Can you work these out from the drawing? Everything is in mm from the part's minimum corner. A direction names the side the tool comes from. Coordinates: 2 decimals unless noted, no trailing zeros. Write each loop counter-clockwise with the first axis right and the second up, starting at its lowest first coordinate (ties: lowest second). Pieces come first, ordered by that corner, then holes. Notation, with made-up numbers: M 69,37.5 L 123,37.5 A25 cw 123,52.5 Z; hole C 74.5,55.5 d4. An arc over 180 degrees is marked long. Write item = value, one per line.
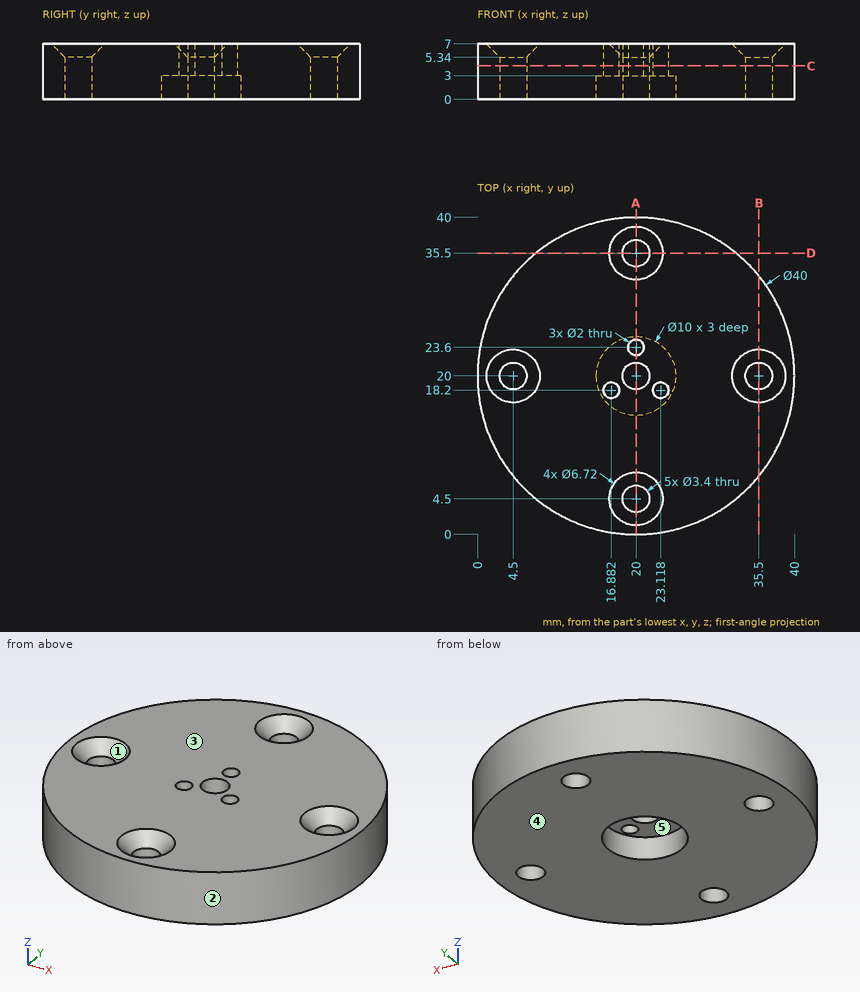
Item 1: Imagine slicing it at C-C (z = 4.25). State how many separate pieces and enclosed holes the cut face has, and give its area (3 significant figures).
Numbers:
separate_pieces = 1
enclosed_holes = 8
area = 1,200 mm²
Item 2: Imagine slicing it at B-B (x = 35.5). Write out the boundary of the cut face in (y, z).
Numbers:
outline = M 7.36,0 L 18.3,0 L 18.3,5.34 L 16.64,7 L 7.36,7 Z; M 21.7,0 L 32.64,0 L 32.64,7 L 23.36,7 L 21.7,5.34 Z
Item 3: If we mould it in two halves opening along Y, with no side actions, what happens to the marked faces 1, 2 and 3? For each: pulls with the +Y half, pulls with the -Y half, needs draft (parallel to the pull), parting line crosses it, or undercut.
Numbers:
face_1 = undercut
face_2 = parting line crosses it
face_3 = needs draft
Item 4: I'm going to push flat-ended pins straight in: P1, Ø4, axis at y = 15, z = 2, coming from the +X side; P2, Ø1, axis at x = 28, z = 3.5, coming from the +Y side. Where does each tip first touch, or does it pass through?
Numbers:
P1 = 39.77
P2 = 38.54
Item 5: Imagine slicing it at A-A (x = 20). Write out the boundary of the cut face in (y, z).
Numbers:
outline = M 0,0 L 2.8,0 L 2.8,5.34 L 1.14,7 L 0,7 Z; M 6.2,0 L 15,0 L 15,3 L 18.3,3 L 18.3,7 L 7.86,7 L 6.2,5.34 Z; M 21.7,3 L 22.6,3 L 22.6,7 L 21.7,7 Z; M 24.6,3 L 25,3 L 25,0 L 33.8,0 L 33.8,5.34 L 32.14,7 L 24.6,7 Z; M 37.2,0 L 40,0 L 40,7 L 38.86,7 L 37.2,5.34 Z
Item 6: For the marked faces 4 and 5, which set-ups out of +Z, -Z, +X, -X, +Y, -Y let a thin tool reach every point of the face, with its end or its side?
Numbers:
face_4 = -Z, +X, -X, +Y, -Y
face_5 = -Z
Item 7: If I drill on line 1 along Y through (x, z) = (20, 2.2); line 2 along Y through (x, z) = (21, 2.5) (1 decimal); line 3 along X through (y, z) = (18, 4.75), over which ranges is the centre line in solid material (lowest first)?
Numbers:
line_1 = 0 to 2.8, 6.2 to 15, 25 to 33.8, 37.2 to 40
line_2 = 0 to 3.1, 5.9 to 15.1, 24.9 to 34.1, 36.9 to 40
line_3 = 0.1 to 15.9, 17.86 to 22.14, 24.1 to 39.9
